Check sheet for the modelled part. Datum: model origin and axes. Units: mm. A direction names the side the tool comes from. Round coordinates to 2 decimals unless told otherwise and drop trailing zeros. Write each loop counter-clockwise with the first axis right and the second up, starting at its lowest first coordinate (ties: lowest second). Pieces come first, ordered by that corner, then holes. Notation, with made-up numbers: (44.5, -36) -> (72.5, -36) arc R15 cw to (72.5, -10) -> close; hole circle Ø3 at (-38.75, -19). An arc over 180 degrees is marked (long way). One line per item, written item: value.
from build123d import *

# Parameters (mm, degrees)
F0_W     = 104.2701750994
F0_H     = 52.628479898
F0_W_2   = 18.0910397321
F0_H_2   = 24.7193295509
F0_W_3   = 17.7621119656
F0_W_4   = 16.775328666
F0_H_3   = 24.3904013187
F1_DEPTH = 8.128
F2_W     = 1.5516094863
F2_H     = 50.6867542863
F2_W_2   = 2.5433897972
F3_DEPTH = 25.4
F4_W     = 21.5143151581
F4_H     = 21.6306117363
F6_DEPTH = 2.286
F5_W     = 21.539459005
F5_H     = 21.8509552069
F7_DEPTH = 2.286


with BuildPart() as f1:
    # F0 (on Top) → F1 (new body)
    with BuildSketch(Plane.XY):
        with Locations((4.019651562, 11.5622095764)):
            Rectangle(F0_W, F0_H)
        with Locations((-26.5706507489, 12.3596647754)):
            Rectangle(F0_W_2, F0_H_2, mode=Mode.SUBTRACT)
        with Locations((2.2105479147, 12.3596647754)):
            Rectangle(F0_W_3, F0_H_2, mode=Mode.SUBTRACT)
        with Locations((35.5967376381, 12.1952006593)):
            Rectangle(F0_W_4, F0_H_3, mode=Mode.SUBTRACT)
    extrude(amount=F1_DEPTH)

    # F2 (on face) → F3 (join)
    with BuildSketch(Plane.XY.offset(8.128)):
        with Locations((-47.3396312445, 10.5913467705)):
            Rectangle(F2_W, F2_H)
        with Locations((54.8830442131, 10.5913467705)):
            Rectangle(F2_W_2, F2_H)
    extrude(amount=F3_DEPTH)

    # F4 (on face) → F6 (join)
    with BuildSketch(Plane.YZ.offset(56.1547391117)):
        with Locations((10.7571575791, 16.2811053451)):
            Rectangle(F4_W, F4_H)
    extrude(amount=F6_DEPTH)

    # F5 (on face) → F7 (join)
    with BuildSketch(Plane(origin=(-48.1154359877, 0, 0), x_dir=(0, -1, 0), z_dir=(-1, 0, 0))):
        with Locations((-10.7697295025, 16.3343714084)):
            Rectangle(F5_W, F5_H)
    extrude(amount=F7_DEPTH)


solid = f1.part
Item 1: Depth check by flat-ended pin: pin 1 (0.7 mm diameter, centred on x = -48.5, z = 14, fed in from -Y); pin 2 (12 mm diameter, centred on y = -9, z = 30, fed in from +X); pin 3 (3 mm diameter, centred on x = 27, y = -8.5, fed in from +Z). Enter the tip coordinate at first touch or a pass-through.
Result set:
pin 1: y = 0
pin 2: x = 56.15
pin 3: z = 8.13
Item 2: Sectioned sample at A-A (x = 30.5). Enter the section's corners in (y, z), then the cut area to 3 significant figures.
Result set:
outline: (-14.75, 0) -> (0, 0) -> (0, 8.13) -> (-14.75, 8.13) -> close; (24.39, 0) -> (37.88, 0) -> (37.88, 8.13) -> (24.39, 8.13) -> close
area: 230 mm^2
Item 3: Sectioned sample at D-D (z = 20.5). Enter the section's corners in (x, y).
Result set:
outline: (-50.4, 0) -> (-48.12, 0) -> (-48.12, -14.75) -> (-46.56, -14.75) -> (-46.56, 35.93) -> (-48.12, 35.93) -> (-48.12, 21.54) -> (-50.4, 21.54) -> close; (53.61, -14.75) -> (56.15, -14.75) -> (56.15, 0) -> (58.44, 0) -> (58.44, 21.51) -> (56.15, 21.51) -> (56.15, 35.93) -> (53.61, 35.93) -> close
Item 4: Release check for a two-part mould opening along Y. For faces 4 (the flat face through (55, 35.935, 21)), 5 (the flat face through (-46.564, 10, 21)), 6 (the flat face through (-27, 0, 4)) record: pulls with the +Y half, pulls with the -Y half, needs draft (parallel to the pull), parting line crosses it, or undercut.
Result set:
face 4: pulls with the +Y half
face 5: needs draft
face 6: undercut
Item 5: Sectioned sample at B-B (z = 7). Enter the section's corners in (x, y).
Result set:
outline: (-50.4, 0) -> (-48.12, 0) -> (-48.12, -14.75) -> (56.15, -14.75) -> (56.15, 0) -> (58.44, 0) -> (58.44, 21.51) -> (56.15, 21.51) -> (56.15, 37.88) -> (-48.12, 37.88) -> (-48.12, 21.54) -> (-50.4, 21.54) -> close; hole (-35.62, 0) -> (-17.53, 0) -> (-17.53, 24.72) -> (-35.62, 24.72) -> close; hole (-6.67, 0) -> (11.09, 0) -> (11.09, 24.72) -> (-6.67, 24.72) -> close; hole (27.21, 0) -> (43.98, 0) -> (43.98, 24.39) -> (27.21, 24.39) -> close
Item 6: Sectioned sample at C-C (y = 8). Enter the section's corners in (x, z), then the cut area to 3 significant figures.
Result set:
outline: (-50.4, 5.41) -> (-48.12, 5.41) -> (-48.12, 0) -> (-35.62, 0) -> (-35.62, 8.13) -> (-46.56, 8.13) -> (-46.56, 33.53) -> (-48.12, 33.53) -> (-48.12, 27.26) -> (-50.4, 27.26) -> close; (-17.53, 0) -> (-6.67, 0) -> (-6.67, 8.13) -> (-17.53, 8.13) -> close; (11.09, 0) -> (27.21, 0) -> (27.21, 8.13) -> (11.09, 8.13) -> close; (43.98, 0) -> (56.15, 0) -> (56.15, 5.47) -> (58.44, 5.47) -> (58.44, 27.1) -> (56.15, 27.1) -> (56.15, 33.53) -> (53.61, 33.53) -> (53.61, 8.13) -> (43.98, 8.13) -> close
area: 623 mm^2
Item 7: Material ranges on line 1 along X through (y, z) = (12, 11); line 2 along X through (y, z) = (2, 8); line 3 along Y through (x, z) = (3.5, 2.5), recorded low to high.
Result set:
line 1: -50.4 to -46.56, 53.61 to 58.44
line 2: -50.4 to -35.62, -17.53 to -6.67, 11.09 to 27.21, 43.98 to 58.44
line 3: -14.75 to 0, 24.72 to 37.88
Item 8: Tool access check on faces 1 (the flat face through (57, 11, 5.466)), 2 (the flat face through (-6.671, 12, 4)), 3 (the flat face through (-49, 0, 16)). Record the directions out of +Z, -Z, +X, -X, +Y, -Y that give a thin tool (end or side, any length) a straight path to the whole face; none if there is none.
Result set:
face 1: -Z, +X, +Y, -Y
face 2: +Z, -Z
face 3: +Z, -Z, -X, -Y
